Part model, mm, in its own coordinate system. Face numbers are marked on the shaded views. A direction names the side the tool comes from. Coordinates: 2 decimals unless noted, no trailing zeros. Order: outer loops, then holes, each group sorted by start corner. A loop starts at its lowest first (then second) coordinate and runs counter-clockwise, first axis right, second up.
1) Cut at D-D (z = -8). List the corners of the cut face in (x, y), and give its area (3 significant figures).
2) Cut at A-A (x = 43). List the corners of the cut face in (y, z), and give its area (3 significant figures).
3) Cut at B-B (y = 1.5). List the corners of the cut face in (x, z) (3 decimals).
4) Mould opens along X. For the marked faces 4, 5, 6 and 7 say: +X half, -X half, draft (parallel to the pull), parting line (faces both ways), or undercut.
5) Tool access for the marked faces 1, 2 and 3: list every direction of +Z, -Z, +X, -X, +Y, -Y with a clear straight run to the whole face (end or side of a thin tool).
6) Cut at C-C (y = -2). Give the number of separate pieces and of enclosed holes in the cut face, and give its area (3 significant figures).
7) Pin check, flat tips, straight feed: pin 1 Ø5 at (y, z) = (3.5, 1) entering from -X; pin 2 Ø5 at (x, y) = (26, 1.5) entering from -Z; pin 3 Ø5 at (x, y) = (37.5, -3) entering from -Z. Stop position of each tip, or through.
8) Wall check: L1, parallel to Y at x = 21.5, z = -2; L2, parallel to Z at x = 24, y = -0.75; L3, parallel to Z at x = 56, y = -2.5. Give the ranges that are in metal, low to high.
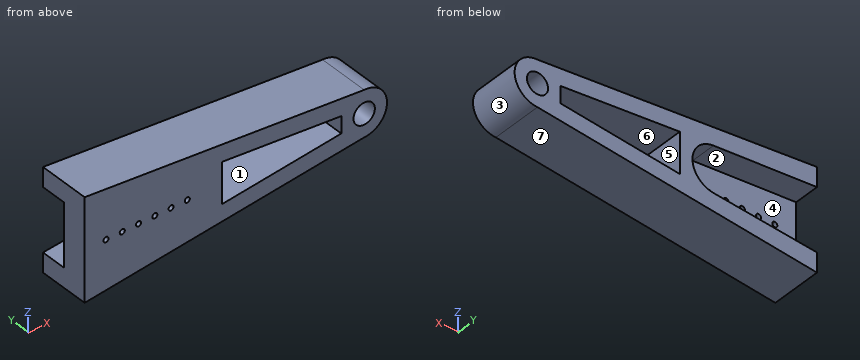
```python
from build123d import *

# Parameters (mm, degrees)
SKETCH1_R               = 2.075
BOSS_EXTRUDE1_DEPTH     = 5
BOSS_EXTRUDE4_START     = -5
SKETCH4_R               = 0.5
SKETCH4_R_2             = 2.1
BOSS_EXTRUDE4_DEPTH     = 5
CUT_EXTRUDE1_DEPTH      = 5
CUT_EXTRUDE1_DEPTH_BACK = 5


with BuildPart() as part:
    # Sketch1 → Boss-Extrude1 (new body)
    with BuildSketch(Plane(origin=(0, 0, 0), x_dir=(1, 0, 0), z_dir=(0, 1, 0))):
        with BuildLine():
            Line((10, 6.188190874), (30.375, 4.484347779))
            ThreePointArc((30.375, 4.484347779), (34.5, 0), (30.375, -4.484347779))
            Line((30.375, -4.484347779), (10, -6.188190874))
            Line((10, -6.188190874), (10, -10))
            Line((10, -10), (65, -4.5))
            ThreePointArc((65, -4.5), (69.5, 0), (65, 4.5))
            Line((65, 4.5), (10, 10))
            Line((10, 10), (10, 6.188190874))
        make_face()
        with Locations(Location((65, 0, 0), (0, 0, 270))):
            Circle(SKETCH1_R, mode=Mode.SUBTRACT)
    extrude(amount=BOSS_EXTRUDE1_DEPTH)

    # Sketch4 → Boss-Extrude4 (add)
    with BuildSketch(Plane(origin=(0, 0, 0), x_dir=(1, 0, 0), z_dir=(0, 1, 0)).offset(BOSS_EXTRUDE4_START)):
        with BuildLine():
            Line((10, 10), (10, -10))
            Line((10, -10), (65, -4.5))
            ThreePointArc((65, -4.5), (69.5, 0), (65, 4.5))
            Line((65, 4.5), (10, 10))
        make_face()
        with Locations(Location((14.2, 0, 0), (0, 0, 270))):
            Circle(SKETCH4_R, mode=Mode.SUBTRACT)
        with Locations(Location((17.4, 0, 0), (0, 0, 270))):
            Circle(SKETCH4_R, mode=Mode.SUBTRACT)
        with Locations(Location((20.6, 0, 0), (0, 0, 270))):
            Circle(SKETCH4_R, mode=Mode.SUBTRACT)
        with Locations(Location((23.8, 0, 0), (0, 0, 270))):
            Circle(SKETCH4_R, mode=Mode.SUBTRACT)
        with Locations(Location((27, 0, 0), (0, 0, 270))):
            Circle(SKETCH4_R, mode=Mode.SUBTRACT)
        with Locations(Location((30.2, 0, 0), (0, 0, 270))):
            Circle(SKETCH4_R, mode=Mode.SUBTRACT)
        with Locations(Location((65, 0, 0), (0, 0, 270))):
            Circle(SKETCH4_R_2, mode=Mode.SUBTRACT)
    extrude(amount=BOSS_EXTRUDE4_DEPTH)

    # Sketch3 → Cut-Extrude1 (cut, two sides: drawn at the far end of the back side and taken through both)
    with BuildSketch(Plane(origin=(0, 0, 0), x_dir=(1, 0, 0), z_dir=(0, 1, 0)).offset(-CUT_EXTRUDE1_DEPTH_BACK)):
        Polygon((60.5, -1.65), (60.5, 1.65), (37, 4), (37, -4), align=None)
    extrude(amount=CUT_EXTRUDE1_DEPTH + CUT_EXTRUDE1_DEPTH_BACK, mode=Mode.SUBTRACT)


solid = part.part
```
Geometry check:
1. outline: (10, -5) - (30, -5) - (30, 5) - (10, 5) - close
1. area: 200 mm2
2. outline: (-5, -6.7) - (5, -6.7) - (5, -3.4) - (-5, -3.4) - close; (-5, 3.4) - (5, 3.4) - (5, 6.7) - (-5, 6.7) - close
2. area: 66.0 mm2
3. outline: (10, -10) - (65, -4.5) arc R4.5 ccw to (65, 4.5) - (10, 10) - (10, 6.188) - (30.375, 4.484) arc R4.5 cw to (30.375, -4.484) - (10, -6.188) - close; hole (37, -4) - (60.5, -1.65) - (60.5, 1.65) - (37, 4) - close; hole circle Ø4.15 at (65, 0)
4. face 4: draft
4. face 5: undercut
4. face 6: undercut
4. face 7: +X half
5. face 1: +Y, -Y
5. face 2: -X, +Y
5. face 3: +X, +Y, -Y
6. separate pieces: 1
6. enclosed holes: 8
6. area: 678 mm2
7. pin 1: stops at x = 32.83
7. pin 2: stops at z = -8.65
7. pin 3: stops at z = -7.5
8. L1: y = -5 to 0
8. L2: z = -8.6 to -0.46, 0.46 to 8.6
8. L3: z = -5.4 to -2.1, 2.1 to 5.4
